Here's how the part is built. I have some questions about the finished solid (model axes, mm). Round coordinates to 2 decimals unless told otherwise and drop trailing zeros. Loops run counter-clockwise (first coordinate to the right, second up) from the corner with the lowest first, then second, coordinate; pieces in that order, holes last. Notation, with made-up numbers: (-39.5, 49) - (4.5, 49) arc R26 cw to (4.5, 66) - close; hole circle Ø9 at (50, 89). An arc over 180 degrees is marked (long way). Return JSON: item names as keys, results as strings. Group by question number.
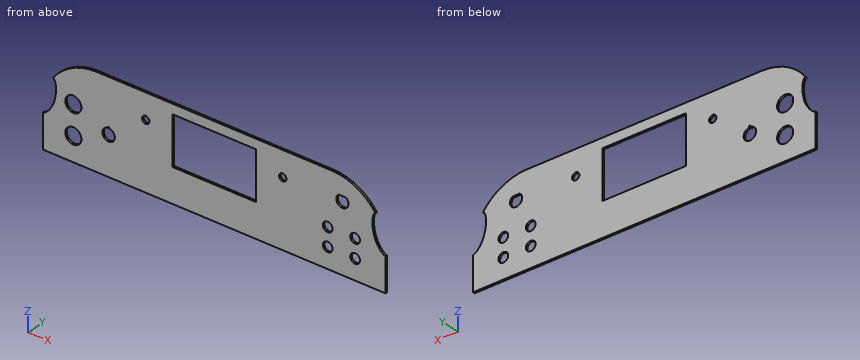
```python
from build123d import *

# Parameters (mm, degrees)
BOSS_EXTRUDE1_DEPTH = 2.54
SKETCH2_W           = 107.95
SKETCH2_H           = 63.5
CUT_EXTRUDE1_DEPTH  = 238.771783963
CUT_EXTRUDE4_REACH  = 239.772
SKETCH4_R           = 4.7625
SKETCH4_R_2         = 6.35
SKETCH4_R_3         = 10.5
CUT_EXTRUDE3_DEPTH  = 238.771784093


with BuildPart() as part:
    # Sketch1 → Boss-Extrude1 (new body)
    with BuildSketch(Plane(origin=(0, 0, 0), x_dir=(1, 0, 0), z_dir=(0, 1, 0))):
        with BuildLine():
            Line((222.25, -14.612459999), (222.25, 36.187540001))
            Line((222.25, 36.187540001), (-222.25, 36.187540001))
            Line((-222.25, 36.187540001), (-222.25, -14.612459999))
            ThreePointArc((-222.25, -14.612459999), (-201.791408666, -64.003868664), (-152.4, -84.462459999))
            Line((-152.4, -84.462459999), (152.4, -84.462459999))
            ThreePointArc((152.4, -84.462459999), (201.791408666, -64.003868664), (222.25, -14.612459999))
        make_face()
    extrude(amount=BOSS_EXTRUDE1_DEPTH)

    # Sketch2 → Cut-Extrude1 (cut, through all)
    with BuildSketch(Plane(origin=(0, 2.54, 0), x_dir=(1, 0, 0), z_dir=(0, 1, 0))):
        with Locations((0, -40.012459999)):
            Rectangle(SKETCH2_W, SKETCH2_H)
    extrude(amount=-CUT_EXTRUDE1_DEPTH, mode=Mode.SUBTRACT)

    # Sketch5 → Cut-Extrude4 (cut, up to next)
    with BuildSketch(Plane(origin=(0, 2.54, 0), x_dir=(1, 0, 0), z_dir=(0, 1, 0)), mode=Mode.PRIVATE) as cut_extrude4_sk1:
        with BuildLine():
            ThreePointArc((-222.25, -14.612459999), (-218.970589391, -35.763798683), (-209.440289817, -54.929055063))
            add(Edge.make_bspline(
                [(-209.440289817, -54.929055063), (-204.823931799, -55.506078622), (-202.304901657, -25.266816537), (-219.26819847, -8.373976847), (-222.25, -8.829558466)],
                knots=[0, 0, 0, 0, 0.32580352, 0.516674914, 0.516674914, 0.516674914, 0.516674914], degree=3))
            Line((-222.25, -8.829558466), (-222.25, -14.612459999))
        make_face()
    cut_extrude4_tool1 = extrude(cut_extrude4_sk1.sketch, amount=-CUT_EXTRUDE4_REACH, mode=Mode.PRIVATE) & part.part
    # Sketch5 → Cut-Extrude4 (cut, up to next)
    with BuildSketch(Plane(origin=(0, 2.54, 0), x_dir=(1, 0, 0), z_dir=(0, 1, 0)), mode=Mode.PRIVATE) as cut_extrude4_sk2:
        with BuildLine():
            add(Edge.make_bspline(
                [(209.440289817, -54.929055063), (204.823931799, -55.506078622), (202.304901657, -25.266816537), (235.136564978, 7.428480335), (216.288594077, -54.073048471), (209.440289817, -54.929055063)],
                knots=[0, 0, 0, 0, 0.32580352, 0.516674914, 1, 1, 1, 1], degree=3))
        make_face()
    cut_extrude4_tool2 = extrude(cut_extrude4_sk2.sketch, amount=-CUT_EXTRUDE4_REACH, mode=Mode.PRIVATE) & part.part
    add(cut_extrude4_tool1.solids().sort_by_distance((-213.6132, 2.54, 31.506825))[0], mode=Mode.SUBTRACT)
    add(cut_extrude4_tool2.solids().sort_by_distance((214.431319, 2.54, 31.263671))[0], mode=Mode.SUBTRACT)

    # Sketch4 → Cut-Extrude3 (cut, through all)
    with BuildSketch(Plane(origin=(0, 2.54, 0), x_dir=(1, 0, 0), z_dir=(0, 1, 0))):
        with Locations(Location((88.9, -51.442459999, 0), (0, 0, 270))):
            Circle(SKETCH4_R)
        with Locations(Location((147.32, -14.612459999, 0), (0, 0, 270))):
            Circle(SKETCH4_R_2)
        with Locations(Location((147.32, 9.517540001, 0), (0, 0, 270))):
            Circle(SKETCH4_R_2)
        with Locations(Location((182.88, 9.517540001, 0), (0, 0, 270))):
            Circle(SKETCH4_R_2)
        with Locations(Location((-88.9, -51.442459999, 0), (0, 0, 270))):
            Circle(SKETCH4_R)
        with Locations(Location((-182.88, -33.662459999, 0), (0, 0, 270))):
            Circle(SKETCH4_R_3)
        with Locations(Location((-182.88, 4.437540001, 0), (0, 0, 270))):
            Circle(SKETCH4_R_3)
        with Locations(Location((182.88, -14.612459999, 0), (0, 0, 270))):
            Circle(SKETCH4_R_2)
        with BuildLine():
            Line((-138.01, -22.667737772), (-138.01, -24.412459999))
            Line((-138.01, -24.412459999), (-136.31, -24.412459999))
            Line((-136.31, -24.412459999), (-136.31, -22.667737772))
            ThreePointArc((-136.31, -22.667737772), (-137.16, -6.512459999), (-138.01, -22.667737772))
        make_face()
        with BuildLine():
            Line((171.1325, -59.062459999), (161.6075, -59.062459999))
            ThreePointArc((161.6075, -59.062459999), (166.37, -44.774959999), (171.1325, -59.062459999))
        make_face()
    extrude(amount=-CUT_EXTRUDE3_DEPTH, mode=Mode.SUBTRACT)


solid = part.part
```
Q1. Imagine slicing it at B-B, the plane x = 147.32. List the corners of the cut face in (y, z) for me, and give its area (3 significant figures).
Q2. Imagine slicing it at D-D, the plane x = 88.9. List the corners of the cut face in (y, z) for me, and give its area (3 significant figures).
Q3. Please list where these lines run through material, in increasing order: line 1 (X direction, y = 0.75, z = 17) (3 decimals); line 2 (Z direction, x = 46.5, y = 2.4); line 3 (X direction, y = 2.05, z = -4).
Q4. Imagine slicing it at C-C, the plane y = 1.75. Give the number of separate pieces and of enclosed holes in the cut face, and give its area (3 significant figures).
Q5. Imagine slicing it at A-A, the plane x = -48. List the corners of the cut face in (y, z) for me.
Q6. Will these pins go through, and if not, where does the flat tip stop? pin 1 Ø14.5 at (x, z) = (-137.16, 14.61) entering from -Y; pin 2 Ø1.4 at (y, z) = (1.5, 24) entering from -X; pin 3 Ø0.5 at (y, z) = (0.5, 24) entering from +X; pin 4 Ø1.3 at (y, z) = (1.5, 41) entering from +X.
Output values:
{
 "1": {"outline": "(0, -36.19) - (2.54, -36.19) - (2.54, -15.87) - (0, -15.87) - close; (0, -3.17) - (2.54, -3.17) - (2.54, 8.26) - (0, 8.26) - close; (0, 20.96) - (2.54, 20.96) - (2.54, 84.46) - (0, 84.46) - close", "area": "242 mm^2"},
 "2": {"outline": "(0, -36.19) - (2.54, -36.19) - (2.54, 46.68) - (0, 46.68) - close; (0, 56.2) - (2.54, 56.2) - (2.54, 84.46) - (0, 84.46) - close", "area": "282 mm^2"},
 "3": {"line 1": "x = -212.537 to -144.9, -129.42 to -53.975, 53.975 to 141.436, 153.204 to 176.996, 188.764 to 212.537", "line 2": "z = -36.19 to 8.26, 71.76 to 84.46", "line 3": "x = -222.25 to -193.37, -172.39 to 144.18, 150.46 to 179.74, 186.02 to 222.25"},
 "4": {"separate pieces": "1", "enclosed holes": "11", "area": "42,000 mm^2"},
 "5": {"outline": "(0, -36.19) - (2.54, -36.19) - (2.54, 8.26) - (0, 8.26) - close; (0, 71.76) - (2.54, 71.76) - (2.54, 84.46) - (0, 84.46) - close"},
 "6": {"pin 1": "passes through", "pin 2": "stops at x = -209.12", "pin 3": "stops at x = 208.93", "pin 4": "stops at x = 205.41"}
}
